```python
from build123d import *

# Parameters (mm, degrees)
SKETCH_2_W           = 14
SKETCH_2_H           = 14
EXTRUDE_1_DEPTH      = 1.4
SKETCH_1_W           = 13.5
SKETCH_1_H           = 13.5
SKETCH_8_W           = 15.5
SKETCH_8_H           = 15.5
EXTRUDE_2_DEPTH      = 1
SKETCH_10_W          = 10
SKETCH_10_H          = 9.5
SKETCH_12_W          = 7
SKETCH_12_H          = 5
EXTRUDE_3_DEPTH      = 0.5
EXTRUDE_5_DEPTH      = 4
SKETCH_16_R          = 2
EXTRUDE_6_DEPTH      = 3
CHAMFER_1_SIZE       = 0.25
CHAMFER_1_SIZE2      = 0.686869355
SKETCH_18_W          = 8
SKETCH_18_H          = 3
CUT_EXTRUDE_1_DEPTH  = 4.5
SKETCH_20_W          = 2.183812488
SKETCH_20_H          = 3.542412762
CUT_EXTRUDE_9_DEPTH  = 5
SKETCH_23_W          = 2.16
SKETCH_23_H          = 4.720066995
CUT_EXTRUDE_10_DEPTH = 5
SKETCH_26_R          = 1.5
CUT_EXTRUDE_12_DEPTH = 5.5
SKETCH_27_W          = 1
SKETCH_27_H          = 0.5
EXTRUDE_7_DEPTH      = 3
CHAMFER_2_SIZE       = 0.25
CHAMFER_2_SIZE2      = 0.686869355
CHAMFER_3_SIZE       = 0.25
CHAMFER_3_SIZE2      = 0.686869355
FILLET_1_R           = 1


with BuildPart() as part:
    # 草图2 → 凸台-拉伸1 (new body)
    with BuildSketch(Plane(origin=(0, 4.5, 0), x_dir=(1, 0, 0), z_dir=(0, 1, 0))):
        Rectangle(SKETCH_2_W, SKETCH_2_H)
    extrude(amount=-EXTRUDE_1_DEPTH)

    # 草图1 → section 1 of loft_2
    with BuildSketch(Plane(origin=(0, 0, 0), x_dir=(1, 0, 0), z_dir=(0, 1, 0)), mode=Mode.PRIVATE) as loft_2_s1:
        Rectangle(SKETCH_1_W, SKETCH_1_H)
    # loft from a face of the part (loft_2)
    loft([part.faces().sort_by_distance((0, 3.1, 0))[0], loft_2_s1.sketch])

    # 草图8 → 凸台-拉伸2 (add)
    with BuildSketch(Plane(origin=(0, 4.5, 0), x_dir=(1, 0, 0), z_dir=(0, 1, 0))):
        Rectangle(SKETCH_8_W, SKETCH_8_H)
    extrude(amount=EXTRUDE_2_DEPTH)

    # 草图10 → section 1 of loft_6
    with BuildSketch(Plane(origin=(0, 11, 0), x_dir=(1, 0, 0), z_dir=(0, 1, 0)), mode=Mode.PRIVATE) as loft_6_s1:
        with Locations((0, -0.75)):
            Rectangle(SKETCH_10_W, SKETCH_10_H)
    # loft from a face of the part (loft_6)
    loft([part.faces().sort_by_distance((0, 5.5, 0))[0], loft_6_s1.sketch])

    # 草图12 → 凸台-拉伸3 (add)
    with BuildSketch(Plane(origin=(0, 11, 0), x_dir=(1, 0, 0), z_dir=(0, 1, 0))):
        Rectangle(SKETCH_12_W, SKETCH_12_H)
    extrude(amount=EXTRUDE_3_DEPTH)

    # 草图14 → 凸台-拉伸5 (add)
    with BuildSketch(Plane(origin=(0, 11.5, 0), x_dir=(1, 0, 0), z_dir=(0, 1, 0))):
        Polygon((0.5, -0.5), (2, -0.5), (2, 0.5), (0.5, 0.5), (0.5, 2.008619841), (-0.5, 2.008619841), (-0.5, 0.5), (-2, 0.5), (-2, -0.5), (-0.5, -0.5), (-0.5, -1.991380159), (0.5, -1.991380159), align=None)
    extrude(amount=EXTRUDE_5_DEPTH)

    # 草图16 → 凸台-拉伸6 (add)
    with BuildSketch(Plane(origin=(0, 0, 0), x_dir=(-1, 0, 0), z_dir=(0, -1, 0))):
        Circle(SKETCH_16_R)
    extrude(amount=EXTRUDE_6_DEPTH)

    # 倒角1
    chamfer_1_edges = [part.edges().sort_by_distance(p)[0] for p in [
        (2, -3, 0),
    ]]
    chamfer_1_side = [part.faces().sort_by_distance(p)[0] for p in [
        (0, -3, 0),
    ]]
    chamfer(chamfer_1_edges, length=CHAMFER_1_SIZE, length2=CHAMFER_1_SIZE2, reference=chamfer_1_side[0])

    # 草图18 → 切除-拉伸1 (cut)
    with BuildSketch(Plane(origin=(0, 11, 0), x_dir=(1, 0, 0), z_dir=(0, 1, 0))):
        with Locations((0, 5.5)):
            Rectangle(SKETCH_18_W, SKETCH_18_H)
    extrude(amount=-CUT_EXTRUDE_1_DEPTH, mode=Mode.SUBTRACT)

    # 草图20 → 切除-拉伸9 (cut)
    with BuildSketch(Plane(origin=(0, 11, 0), x_dir=(1, 0, 0), z_dir=(0, 1, 0))):
        with Locations((6.091906244, 5.228793619)):
            Rectangle(SKETCH_20_W, SKETCH_20_H)
        with Locations((-6.091906244, 5.228793619)):
            Rectangle(SKETCH_20_W, SKETCH_20_H)
    extrude(amount=-CUT_EXTRUDE_9_DEPTH, mode=Mode.SUBTRACT)

    # 草图23 → 切除-拉伸10 (cut)
    with BuildSketch(Plane(origin=(0, 11, 0), x_dir=(1, 0, 0), z_dir=(0, 1, 0))):
        with Locations((6.08, -4.90244626)):
            Rectangle(SKETCH_23_W, SKETCH_23_H)
        with Locations((-6.08, -4.90244626)):
            Rectangle(SKETCH_23_W, SKETCH_23_H)
    extrude(amount=-CUT_EXTRUDE_10_DEPTH, mode=Mode.SUBTRACT)

    # 草图26 → 切除-拉伸12 (cut)
    with BuildSketch(Plane(origin=(0, 11, 0), x_dir=(1, 0, 0), z_dir=(0, 1, 0))):
        with Locations((0, 5.526038024)):
            Circle(SKETCH_26_R)
    extrude(amount=-CUT_EXTRUDE_12_DEPTH, mode=Mode.SUBTRACT)

    # 草图27 → 凸台-拉伸7 (add)
    with BuildSketch(Plane(origin=(0, 0, 0), x_dir=(1, 0, 0), z_dir=(0, 1, 0))):
        with Locations((-2.54, -3.91)):
            Rectangle(SKETCH_27_W, SKETCH_27_H)
        with Locations((3.81, -2.54)):
            Rectangle(SKETCH_27_W, SKETCH_27_H)
    extrude(amount=-EXTRUDE_7_DEPTH)

    # 倒角2
    chamfer_2_edges = [part.edges().sort_by_distance(p)[0] for p in [
        (4.31, -3, 2.54),
        (3.31, -3, 2.54),
    ]]
    chamfer_2_side = [part.faces().sort_by_distance(p)[0] for p in [
        (3.81, -3, 2.54),
    ]]
    chamfer(chamfer_2_edges, length=CHAMFER_2_SIZE, length2=CHAMFER_2_SIZE2, reference=chamfer_2_side[0])

    # 倒角3
    chamfer_3_edges = [part.edges().sort_by_distance(p)[0] for p in [
        (-2.04, -3, 3.91),
        (-3.04, -3, 3.91),
    ]]
    chamfer_3_side = [part.faces().sort_by_distance(p)[0] for p in [
        (-2.54, -3, 3.91),
    ]]
    chamfer(chamfer_3_edges, length=CHAMFER_3_SIZE, length2=CHAMFER_3_SIZE2, reference=chamfer_3_side[0])

    # 圆角1
    fillet_1_edges = [part.edges().sort_by_distance(p)[0] for p in [
        (0, 11, 5.5),
    ]]
    fillet(fillet_1_edges, radius=FILLET_1_R)


solid = part.part
```
For this review, take the finished solid that the model builds, in its own axes (mm). A direction names the side the tool comes from. Round coordinates to 2 decimals unless told otherwise and drop trailing zeros. One line per item, written item: value. Start each with the question number.
(1) Wall thickness on line 1 (X direction, y = 4, z = 1); line 2 (Z direction, x = 0, y = 5.85); line 3 (Y direction, x = 1, z = -4.5): over which ranges is each line inside the solid? List them lowest first.
(2) Insertion check: pin 1 (0.7 mm diameter, centred on y = 14, z = 1, fed in from -X); pin 2 (1.6 mm diameter, centred on y = 14, z = 1, fed in from +X); pin 3 (1.7 mm diameter, centred on x = -6.5, y = 8, fed in from +Z); pin 4 (2 mm diameter, centred on y = 6, z = 4, fed in from +X). Each pin has a flat end and moves straight along its axis. Give the tip position at first contact, or say it passes through.
(3) The part is to be moulded in two halves that separate along X. For faces 1 (the flat face through (-6, 8, -3.458)), 2 (the flat face through (-0.5, 13, 1)), 3 (the flat face through (1, 13, -0.5)), 4 (the flat face through (6, 6, 5)), say which applies: released by +X, released by -X, zero draft, split by the parting line, or undercut.
(4) Machinability: for faces 5 (the flat face through (4, -1, 2.79)), 6 (the cylindrical face through (-0.195, 6.058, -7.013)), 7 (the flat face through (1, 13, 0.5)), 8 (the flat face through (-2, 13, 0)), which of the approach directions +Z, -Z, +X, -X, +Y, -Y give a long, thin tool a straight path to every point of the face, cutting with its end or side? Answer none if there is none.
Result:
1. line 1: -7 to 7
1. line 2: -7.51 to -7.03, -4.03 to 7.61
1. line 3: 0 to 5.5
2. pin 1: x = -0.5
2. pin 2: x = 2
2. pin 3: z = 2.54
2. pin 4: x = 7.75
3. face 1: undercut
3. face 2: released by -X
3. face 3: zero draft
3. face 4: undercut
4. face 5: +Z, +X, -X, -Y
4. face 6: +Y
4. face 7: +Z, +X, +Y
4. face 8: +Z, -Z, -X, +Y
